The model under review builds one solid part; all positions refer to its coordinate system, in mm. A direction names the side the tool comes from. Give positions to 0.01 mm unless a question says otherwise; leave off trailing zeros. Loops run counter-clockwise (first coordinate to the right, second up) from the corner with the lowest first, then second, coordinate; pieces in that order, holes last. Notation, with made-up numbers: M 69.25,80 L 88.25,80 A24 ccw 88.25,111 Z; hole C 25.25,34 d2. An arc over 180 degrees is marked long. Put each result on its own line as item: value. Start each with the question number.
```python
from build123d import *

# Parameters (mm, degrees)
F1_W     = 254
F1_H     = 254
F2_DEPTH = 107.188
F3_R     = 5.08
F4_DEPTH = 242.824
F5_W     = 254
F5_H     = 254
F5_R     = 5.08
F6_DEPTH = 107.188
F7_R     = 5.08
F8_DEPTH = 107.188
F9_DEPTH = 543.306


with BuildPart() as f2:
    # F1 (on Top) → F2 (new body)
    with BuildSketch(Plane.XY):
        Rectangle(F1_W, F1_H)
    extrude(amount=F2_DEPTH)

    # F3 (on face) → F4 (join)
    with BuildSketch(Plane.XY.offset(107.188)):
        Circle(F3_R)
    extrude(amount=F4_DEPTH)

    # F5 (on face) → F6 (join)
    with BuildSketch(Plane.XY.offset(350.012)):
        Rectangle(F5_W, F5_H)
        Circle(F5_R, mode=Mode.SUBTRACT)
    extrude(amount=F6_DEPTH)

    # F7 (on face) → F8 (join)
    with BuildSketch(Plane.XY.offset(350.012)):
        Circle(F7_R)
    extrude(amount=F8_DEPTH)

    # F0 (on Top) → F9 (intersect)
    with BuildSketch(Plane.XY):
        with BuildLine():
            Line((0.5588, -73.3578699913), (0.5588, -15.8651620717))
            ThreePointArc((0.5588, -15.8651620717), (7.9375, -13.7481532851), (13.4602333892, -8.4165160315))
            Line((13.4602333892, -8.4165160315), (63.25037898, -37.1628699913))
            Line((63.25037898, -37.1628699913), (63.80917898, -36.195))
            Line((63.80917898, -36.195), (14.0190333892, -7.4486460402))
            ThreePointArc((14.0190333892, -7.4486460402), (15.875, 0), (14.0190333892, 7.4486460402))
            Line((14.0190333892, 7.4486460402), (63.80917898, 36.195))
            Line((63.80917898, 36.195), (63.25037898, 37.1628699913))
            Line((63.25037898, 37.1628699913), (13.4602333892, 8.4165160315))
            ThreePointArc((13.4602333892, 8.4165160315), (7.9375, 13.7481532851), (0.5588, 15.8651620717))
            Line((0.5588, 15.8651620717), (0.5588, 73.3578699913))
            Line((0.5588, 73.3578699913), (-0.5588, 73.3578699913))
            Line((-0.5588, 73.3578699913), (-0.5588, 15.8651620717))
            ThreePointArc((-0.5588, 15.8651620717), (-7.9375, 13.7481532851), (-13.4602333892, 8.4165160315))
            Line((-13.4602333892, 8.4165160315), (-63.25037898, 37.1628699913))
            Line((-63.25037898, 37.1628699913), (-63.80917898, 36.195))
            Line((-63.80917898, 36.195), (-14.0190333892, 7.4486460402))
            ThreePointArc((-14.0190333892, 7.4486460402), (-15.875, 0), (-14.0190333892, -7.4486460402))
            Line((-14.0190333892, -7.4486460402), (-63.80917898, -36.195))
            Line((-63.80917898, -36.195), (-63.25037898, -37.1628699913))
            Line((-63.25037898, -37.1628699913), (-13.4602333892, -8.4165160315))
            ThreePointArc((-13.4602333892, -8.4165160315), (-7.9375, -13.7481532851), (-0.5588, -15.8651620717))
            Line((-0.5588, -15.8651620717), (-0.5588, -73.3578699913))
            Line((-0.5588, -73.3578699913), (0.5588, -73.3578699913))
        make_face()
        with BuildLine():
            ThreePointArc((-0.5588, -5.0491724629), (-3.3887826723, 3.7845147641), (5.08, 0))
            ThreePointArc((5.08, 0), (3.7845147641, -3.3887826723), (0.5588, -5.0491724629))
            ThreePointArc((0.5588, -5.0491724629), (0, -5.08), (-0.5588, -5.0491724629))
        make_face(mode=Mode.SUBTRACT)
        with BuildLine():
            ThreePointArc((0.5588, -5.0491724629), (3.7845147641, -3.3887826723), (5.08, 0))
            ThreePointArc((5.08, 0), (-3.3887826723, 3.7845147641), (-0.5588, -5.0491724629))
            Line((-0.5588, -5.0491724629), (-0.5588, -0.9678699913))
            Line((-0.5588, -0.9678699913), (0.5588, -0.9678699913))
            Line((0.5588, -0.9678699913), (0.5588, -5.0491724629))
        make_face()
        with BuildLine():
            Line((-0.5588, -0.9678699913), (-0.5588, -5.0491724629))
            ThreePointArc((-0.5588, -5.0491724629), (0, -5.08), (0.5588, -5.0491724629))
            Line((0.5588, -5.0491724629), (0.5588, -0.9678699913))
            Line((0.5588, -0.9678699913), (-0.5588, -0.9678699913))
        make_face()
    extrude(amount=F9_DEPTH, mode=Mode.INTERSECT)


solid = f2.part
```
Item 1: Draft analysis for pull direction Y (two halves, no side actions). For faces 1 (the flat face through (-39.26, 22.02, 52.84)), 2 (the flat face through (-39.26, 22.02, 402.86)), 3 (the cylindrical face through (-0.661, 5.037, 226.9)), 4 (the flat face through (0, 0, 457.2)), state which applies: +Y half, -Y half, draft (parallel to the pull), parting line (faces both ways), or undercut.
Item 2: Clearance check with flat-ended pins moving along their axes: pin 1 Ø8 at (x, z) = (25.5, 388) entering from -Y; pin 2 Ø4 at (y, z) = (36, 365) entering from +X; pin 3 Ø17 at (y, z) = (-32, 399) entering from -X; pin 4 Ø17 at (y, z) = (-47, 63.5) entering from +X. State where each tip first meets the part, or that it passes through.
Item 3: Consider section D-D, the plane y = 0. Write out the cut boundary in (x, z) (3 decimals), plus the area to 3 significant figures.
Item 4: Tool access review of faces 5 (the flat face through (39.26, -22.02, 52.84)), 6 (the cylindrical face through (-7.843, 13.802, 402.856)), 7 (the cylindrical face through (7.843, -13.802, 52.844)): name each direction out of +Z, -Z, +X, -X, +Y, -Y from which nothing blocks a thin tool from reaching the whole face with its end or side.
Item 5: To check wall thickness, follow L1, parallel to X at y = -35, z = 80; L2, parallel to X at y = 24, z = 432; L3, parallel to X at y = -50, z = 82. State the ranges of each line that lie inside material, in increasing order. Write a range as [from, to].
Item 6: Consider section A-A, the plane y = 54. Write out the cut boundary in (x, z), plus the area to 3 significant figures.
Item 7: Consider section C-C, the plane x = -31.5. Write out the cut boundary in (y, z), plus the area to 3 significant figures.
Item 8: Consider section B-B, the plane z = 366. Write out the cut boundary in (x, y) (3 decimals), plus the area to 3 significant figures.
Report:
1. face 1: undercut
1. face 2: undercut
1. face 3: parting line
1. face 4: draft
2. pin 1: y = -17.68
2. pin 2: x = 63.81
2. pin 3: x = -63.81
2. pin 4: x = 0.56
3. outline: M -15.875,0 L 15.875,0 L 15.875,107.188 L 5.08,107.188 L 5.08,350.012 L 15.875,350.012 L 15.875,457.2 L -15.875,457.2 L -15.875,350.012 L -5.08,350.012 L -5.08,107.188 L -15.875,107.188 Z
3. area: 9,270 mm²
4. face 5: +Z, -Z, +X
4. face 6: +Z, -Z, +Y
4. face 7: +Z, -Z, -Y
5. L1: [-61.74, -59.5], [-0.56, 0.56], [59.5, 61.74]
5. L2: [-42.69, -40.45], [-0.56, 0.56], [40.45, 42.69]
5. L3: [-0.56, 0.56]
6. outline: M -0.56,0 L 0.56,0 L 0.56,107.19 L -0.56,107.19 Z; M -0.56,350.01 L 0.56,350.01 L 0.56,457.2 L -0.56,457.2 Z
6. area: 240 mm²
7. outline: M -18.83,0 L -17.54,0 L -17.54,107.19 L -18.83,107.19 Z; M -18.83,350.01 L -17.54,350.01 L -17.54,457.2 L -18.83,457.2 Z; M 17.54,0 L 18.83,0 L 18.83,107.19 L 17.54,107.19 Z; M 17.54,350.01 L 18.83,350.01 L 18.83,457.2 L 17.54,457.2 Z
7. area: 553 mm²
8. outline: M -63.809,-36.195 L -63.25,-37.163 L -13.46,-8.417 A15.875 ccw -0.559,-15.865 L -0.559,-73.358 L 0.559,-73.358 L 0.559,-15.865 A15.875 ccw 13.46,-8.417 L 63.25,-37.163 L 63.809,-36.195 L 14.019,-7.449 A15.875 ccw 14.019,7.449 L 63.809,36.195 L 63.25,37.163 L 13.46,8.417 A15.875 ccw 0.559,15.865 L 0.559,73.358 L -0.559,73.358 L -0.559,15.865 A15.875 ccw -13.46,8.417 L -63.25,37.163 L -63.809,36.195 L -14.019,7.449 A15.875 ccw -14.019,-7.449 Z
8. area: 1,180 mm²
